```python
from build123d import *

# Parameters (mm, degrees)
F1_DEPTH       = 6.35
F2_R           = 3.81
F3_DEPTH       = 6.35
F5_D           = 2.032
F5_CSINK_D     = 3.175
F5_CSINK_ANGLE = 82
F7_D           = 2.032


with BuildPart() as f1:
    # F0 (on Top) → F1 (new body)
    with BuildSketch(Plane.XY):
        with BuildLine():
            ThreePointArc((-5.08, 12.7), (-3.5921024484, 9.1078975516), (0, 7.62))
            Line((0, 7.62), (0, 12.7))
            Line((0, 12.7), (0, 17.78))
            ThreePointArc((0, 17.78), (-3.5921024484, 16.2921024484), (-5.08, 12.7))
        make_face()
        with BuildLine():
            Line((0, 12.7), (0, 7.62))
            ThreePointArc((0, 7.62), (3.5921024484, 9.1078975516), (5.08, 12.7))
            ThreePointArc((5.08, 12.7), (3.5921024484, 16.2921024484), (0, 17.78))
            Line((0, 17.78), (0, 12.7))
        make_face()
        with BuildLine():
            ThreePointArc((5.08, 12.7), (3.5921024484, 9.1078975516), (0, 7.62))
            ThreePointArc((0, 7.62), (-3.5921024484, 9.1078975516), (-5.08, 12.7))
            Line((-5.08, 12.7), (-5.08, 0))
            ThreePointArc((-5.08, 0), (0, -5.08), (5.08, 0))
            Line((5.08, 0), (5.08, 12.7))
        make_face()
        with BuildLine():
            ThreePointArc((0, 17.78), (3.5921024484, 16.2921024484), (5.08, 12.7))
            Line((5.08, 12.7), (5.08, 32.7368881382))
            Line((5.08, 32.7368881382), (4.2115108686, 31.4493000504))
            ThreePointArc((4.2115108686, 31.4493000504), (2.384915539, 29.8046262283), (0, 29.21))
            Line((0, 29.21), (0, 17.78))
        make_face()
        with BuildLine():
            Line((-5.08, 34.29), (-5.08, 12.7))
            ThreePointArc((-5.08, 12.7), (-3.5921024484, 16.2921024484), (0, 17.78))
            Line((0, 17.78), (0, 29.21))
            ThreePointArc((0, 29.21), (-3.5921024484, 30.6978975516), (-5.08, 34.29))
        make_face()
        with BuildLine():
            Line((4.2115108686, 31.4493000504), (5.08, 32.7368881382))
            Line((5.08, 32.7368881382), (5.08, 34.29))
            ThreePointArc((5.08, 34.29), (4.4853737717, 36.674915539), (2.8406999496, 38.5015108686))
            Line((2.8406999496, 38.5015108686), (0, 34.29))
            Line((0, 34.29), (0, 29.21))
            ThreePointArc((0, 29.21), (2.384915539, 29.8046262283), (4.2115108686, 31.4493000504))
        make_face()
        with BuildLine():
            Line((5.08, 34.29), (5.08, 32.7368881382))
            Line((5.08, 32.7368881382), (25.8370032919, 63.5104110421))
            ThreePointArc((25.8370032919, 63.5104110421), (24.466192373, 70.5626218603), (17.4139815548, 69.1918109413))
            Line((17.4139815548, 69.1918109413), (-4.2115108686, 37.1306999496))
            ThreePointArc((-4.2115108686, 37.1306999496), (-0.9693096965, 39.2766660919), (2.8406999496, 38.5015108686))
            ThreePointArc((2.8406999496, 38.5015108686), (4.4853737717, 36.674915539), (5.08, 34.29))
        make_face()
        with BuildLine():
            ThreePointArc((-4.2115108686, 37.1306999496), (-4.8580281603, 35.77524826), (-5.08, 34.29))
            ThreePointArc((-5.08, 34.29), (-3.5921024484, 30.6978975516), (0, 29.21))
            Line((0, 29.21), (0, 34.29))
            Line((0, 34.29), (2.8406999496, 38.5015108686))
            ThreePointArc((2.8406999496, 38.5015108686), (-0.9693096965, 39.2766660919), (-4.2115108686, 37.1306999496))
        make_face()
    extrude(amount=F1_DEPTH)

    # F2 (on face) → F3 (join)
    with BuildSketch(Plane.XY.offset(6.35)):
        with Locations((0, 12.7)):
            Circle(F2_R)
    extrude(amount=F3_DEPTH)

    # F5 (through all)
    with Locations(Plane.XY.offset(12.7)):
        with Locations((0, 12.7)):
            CounterSinkHole(F5_D / 2, F5_CSINK_D / 2, counter_sink_angle=F5_CSINK_ANGLE)

    # F7 (through all)
    with Locations(Plane.XY.offset(6.35)):
        with Locations((0, 0)):
            Hole(F7_D / 2)


solid = f1.part
```
Model file for the job. Use its own axes, mm. A direction names the side the tool comes from. Coordinates: 2 decimals unless noted, no trailing zeros. Order: outer loops, then holes, each group sorted by start corner. A loop starts at its lowest first (then second) coordinate and runs counter-clockwise, first axis right, second up. Notation, with made-up numbers: M 62,-1 L 75,-1 A21 ccw 75,38 Z; hole C 8,89.5 d9. An arc over 180 degrees is marked long. Answer as CSV lines item,"result".
(1) Band-saw the part on B-B, the plane z = 1. List the corners of the cut face in (x, y).
Geometry says:
outline,"M -5.08,0 A5.08 ccw 5.08,0 L 5.08,32.74 L 25.84,63.51 A5.08 ccw 17.41,69.19 L -4.21,37.13 A5.08 ccw -5.08,34.29 Z; hole C 0,0 d2.03; hole C 0,12.7 d2.03"
(2) Wall check: line 1 along X through (y, z) = (12.7, 3.25); line 2 along Y through (x, z) = (-0.5, 3.75); line 3 along Y through (x, z) = (0, 5). Give the ranges that are in metal, low to high.
Geometry says:
line 1,"x = -5.08 to -1.02, 1.02 to 5.08"
line 2,"y = -5.06 to -0.88, 0.88 to 11.82, 13.58 to 42.63"
line 3,"y = -5.08 to -1.02, 1.02 to 11.68, 13.72 to 43.37"
(3) Band-saw the part on A-A, the plane y = 12.7. List the corners of the cut face in (x, z), then the cut area to 3 significant figures.
Geometry says:
outline,"M -5.08,0 L -1.02,0 L -1.02,12.04 L -1.59,12.7 L -3.81,12.7 L -3.81,6.35 L -5.08,6.35 Z; M 1.02,0 L 5.08,0 L 5.08,6.35 L 3.81,6.35 L 3.81,12.7 L 1.59,12.7 L 1.02,12.04 Z"
area,"86.7 mm2"
(4) Flat gauge pins, fed straight in: pin 1 (9.5 mm diameter, centred on x = 14.5, y = 16, fed in from +Z); pin 2 (4 mm diameter, centred on x = 11.5, z = 1.5, fed in from -Y); pin 3 (5 mm diameter, centred on x = 19, z = 7.5, fed in from +Y); pin 4 (1 mm diameter, centred on x = 15.5, z = 4, fed in from +Y). Where does each tip first touch, or does it go through?
Geometry says:
pin 1,"passes through"
pin 2,"stops at y = 39.29"
pin 3,"stops at y = 71.41"
pin 4,"stops at y = 67.1"
(5) Pull direction X, two halves, no side cores. Call faces 3 (the cylindrical face through (0.22, -0.99, 3.13)), 4 (the flat face through (5.08, 16, 3)), 5 (the flat face through (5, 36, 6.35)): +X half, -X half, draft (parallel to the pull), parting line (faces both ways), or undercut.
Geometry says:
face 3,"undercut"
face 4,"+X half"
face 5,"draft"
(6) Band-saw the part on C-C, the plane x = 0. List the corners of the cut face in (y, z), then the cut area to 3 significant figures.
Geometry says:
outline,"M -5.08,0 L -1.02,0 L -1.02,6.35 L -5.08,6.35 Z; M 1.02,0 L 11.68,0 L 11.68,12.04 L 11.11,12.7 L 8.89,12.7 L 8.89,6.35 L 1.02,6.35 Z; M 13.72,0 L 43.37,0 L 43.37,6.35 L 16.51,6.35 L 16.51,12.7 L 14.29,12.7 L 13.72,12.04 Z"
area,"317 mm2"
(7) Band-saw the part on D-D, the plane y = 24.5. List the corners of the cut face in (x, z).
Geometry says:
outline,"M -5.08,0 L 5.08,0 L 5.08,6.35 L -5.08,6.35 Z"
(8) 3-axis set-ups, long thin cutter, end or side, ignore diameter. For faces 1 (the cylindrical face through (0.22, 11.71, 5.94)), 2 (the cylindrical face through (-0.83, 8.98, 9.48)): which of +Z, -Z, +X, -X, +Y, -Y reach the whole face in a straight line?
Geometry says:
face 1,"+Z, -Z"
face 2,"+Z"
